Geometry: final body of the model. Coordinates: model frame, mm. Face numbers are marked on the shaded views. A direction names the side the tool comes from. Round coordinates to 2 decimals unless told otherwise and drop trailing zeros. Loops run counter-clockwise (first coordinate to the right, second up) from the corner with the lowest first, then second, coordinate; pieces in that order, holes last. Notation, with made-up numbers: (82.25, -27) - (139.25, -27) arc R15 ccw to (139.25, -21) - close; hole circle Ø2 at (46, -9.5). An arc over 180 degrees is marked (long way). Answer in a Markdown table with one row per item. Add a question column.
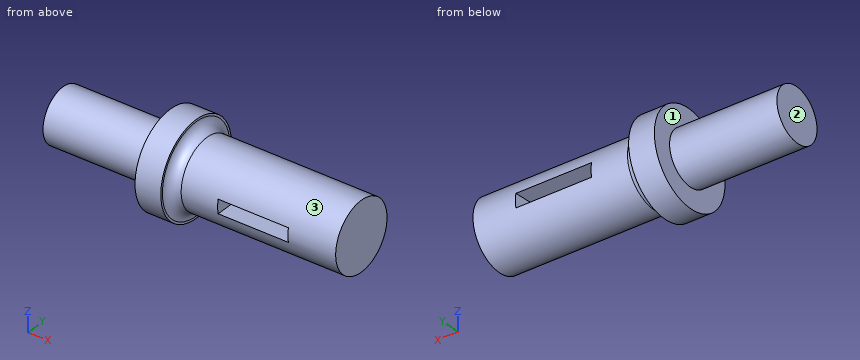
from build123d import *

# Parameters (mm, degrees)
CUT_EXTRUDE1_DEPTH = 3.25


with BuildPart() as part:
    # Sketch1 → Revolve1 (revolve)
    with BuildSketch(Plane(origin=(0, 0, 0), x_dir=(1, 0, 0), z_dir=(0, 1, 0)), mode=Mode.PRIVATE) as revolve1_sk:
        with BuildLine():
            Line((-139, 0), (0, 0))
            Line((0, 0), (0, 16))
            Line((0, 16), (-72, 16))
            ThreePointArc((-72, 16), (-75.535533906, 17.464466094), (-77, 21))
            Line((-77, 21), (-77, 22))
            Line((-77, 22), (-89, 22))
            Line((-89, 22), (-89, 12.5))
            Line((-89, 12.5), (-139, 12.5))
            Line((-139, 12.5), (-139, 0))
        make_face()
    revolve(revolve1_sk.sketch.rotate(Axis((-139, 0, 0), (1, 0, 0)), 180), axis=Axis((-139, 0, 0), (1, 0, 0)))

    # Sketch2 → Cut-Extrude1 (cut, symmetric)
    with BuildSketch(Plane.XY):
        Polygon((-55, 0), (-55, 50), (-17, 50), (-25, -50), (-55, -50), align=None)
    extrude(amount=CUT_EXTRUDE1_DEPTH, both=True, mode=Mode.SUBTRACT)


solid = part.part
1) Section B-B, the plane z = 0. Return the cut outline in (x, y), and give its area (3 significant figures).
2) Material intervals for line 1 along X through (y, z) = (5.5, -2.5); line 2 along X through (y, z) = (-15, -4); line 3 along X through (y, z) = (-6.5, -1.5), sorted ascending. Write a range as from..to.
3) Contact query for flat-ended pins moving along their axis: pin 1 Ø15.5 at (x, y) = (-31.5, 3.5) entering from -Z; pin 2 Ø3 at (x, z) = (-28.5, -14) entering from +Y; pin 3 Ø5 at (x, z) = (-62, 6.5) entering from -Y. Output: stop coordinate, or through.
4) Reachability of the marked faces 1, 2 and 3 from +Z, -Z, +X, -X, +Y, -Y: full face, straight path, thin tool, end or side. Return the list, or none.
5) Section C-C, the plane x = -39.5. Return the cut outline in (y, z).
6) Section A-A, the plane y = 0. Return the cut outline in (x, z).
7) Section D-D, the plane x = -103. Return the cut outline in (y, z).
Evaluation:
| question | item | result |
|---|---|---|
| 1 | outline | (-139, -12.5) - (-89, -12.5) - (-89, -22) - (-77, -22) - (-77, -21) arc R5 cw to (-72, -16) - (-55, -16) - (-55, 16) - (-72, 16) arc R5 cw to (-77, 21) - (-77, 22) - (-89, 22) - (-89, 12.5) - (-139, 12.5) - close; (-22.28, -16) - (0, -16) - (0, 16) - (-19.72, 16) - close |
| 1 | area | 3,160 mm² |
| 2 | line 1 | x = -139..-55, -20.56..0 |
| 2 | line 2 | x = -89..0 |
| 2 | line 3 | x = -139..-55, -21.52..0 |
| 3 | pin 1 | stops at z = -16 |
| 3 | pin 2 | stops at y = 9.99 |
| 3 | pin 3 | stops at y = -15.49 |
| 4 | face 1 | -X |
| 4 | face 2 | +Z, -Z, -X, +Y, -Y |
| 4 | face 3 | +X |
| 5 | outline | (-15.67, -3.25) arc R16 ccw to (15.67, -3.25) - close; (-15.67, 3.25) - (15.67, 3.25) arc R16 ccw to start |
| 6 | outline | (-139, -12.5) - (-89, -12.5) - (-89, -22) - (-77, -22) - (-77, -21) arc R5 cw to (-72, -16) - (0, -16) - (0, 16) - (-72, 16) arc R5 cw to (-77, 21) - (-77, 22) - (-89, 22) - (-89, 12.5) - (-139, 12.5) - close; hole (-55, -3.25) - (-21, -3.25) - (-21, 3.25) - (-55, 3.25) - close |
| 7 | outline | circle Ø25 at (0, 0) |
